Autodesk Inventor part; units mm, degrees
ref_plane "YZ Plane" through (0, 0, 0) normal (1, 0, 0) x (0, 1, 0)
ref_plane "XZ Plane" through (0, 0, 0) normal (0, 1, 0) x (-1, 0, 0)
ref_plane "XY Plane" through (0, 0, 0) normal (0, 0, 1) x (1, 0, 0)
sketch "Sketch1" plane through (0, 0, 0) normal (1, 0, 0) x (0, 1, 0)
  line L0 (24, 0) -> (64, 0)
  line L1 (64, 0) -> (64, 85)
  line L2 (64, 85) -> (24, 85)
  line L3 (24, -2) -> (24, 0)
  line L4 (24, 0) -> (24, 85)
  line L5 (24, 0) -> (109, 0) construction
  point P0 (0, 0)
  dimension "d1" = 85
  dimension "d13" = 90
extrude "Extrusion1" add sketch "Sketch1" along normal blind 2
sketch "Sketch2" plane through (2, 0, 0) normal (1, 0, 0) x (0, 0, -1)
  circle A0 centre (-75.4, 56) radius 1.85
  circle A1 centre (-75.4, 40) radius 1.85
  circle A2 centre (-9.6, 56) radius 1.85
  circle A3 centre (-9.6, 40) radius 1.85
  line L0 (-69, 24) -> (-69, 64)
  line L1 (-16, 24) -> (-16, 64)
  line L2 (-16, 0) -> (48, 0) construction
  line L3 (-85, 64) -> (-85, 24)
  line L4 (-69, 64) -> (-85, 64)
  line L5 (-85, 64) -> (-85, 24)
  line L6 (-69, 24) -> (-69, 64)
  line L7 (0, 24) -> (0, 64)
  line L8 (-16, 64) -> (0, 64)
  line L9 (0, 64) -> (0, 24)
  line L10 (-16, 24) -> (-16, 64)
  line L11 (-85, 24) -> (0, 24)
  point P0 (-69, 0)
  dimension "d5" = 90
extrude "Extrusion2" add sketch "Sketch2" along normal blind 3.2
chamfer "Chamfer1" distance 3.175 angle 45 2 edges at (2, 44, 16) (2, 44, 69)
sketch "Sketch3" plane through (5.2, 0, 0) normal (1, 0, 0) x (0, 0, -1)
  circle A0 centre (-75.4, 56) radius 1.85
  circle A1 centre (-75.4, 40) radius 1.85
  circle A2 centre (-9.6, 40) radius 1.85
  circle A3 centre (-9.6, 56) radius 1.85
  point P0 (0, 0)
extrude "Extrusion3" cut sketch "Sketch3" against normal through all
properties part number "wheelguard"
Can you work these out from the model? Positions are in its coordinate system, mm. A direction names the side the tool comes from. Give positions to 0.01 mm unless a question says otherwise; leave off trailing zeros. Write each loop counter-clockwise with the first axis right and the second up, starting at its lowest first coordinate (ties: lowest second). Pieces come first, ordered by that corner, then holes. Notation, with made-up numbers: (-29, 25) -> (25, 25) arc R11 ccw to (25, 36) -> close; hole circle Ø4 at (88, 19). An arc over 180 degrees is marked (long way). Write item = value, one per line.
(1) Suppose I cut it at A-A on x = 3.6. Write out the boundary of the cut face in (y, z) (3 decimals).
Worked out:
outline = (24, 0) -> (64, 0) -> (64, 17.575) -> (24, 17.575) -> close; (24, 67.425) -> (64, 67.425) -> (64, 85) -> (24, 85) -> close; hole circle Ø3.7 at (40, 9.6); hole circle Ø3.7 at (40, 75.4); hole circle Ø3.7 at (56, 9.6); hole circle Ø3.7 at (56, 75.4)
(2) Thinking about a two-plate mould opening in Z: for faces 1 (the face through (3, 44, 85)), 2 (the face through (0, 44, 43)), 3 (the face through (3.61, 43.72, 17.565)), which applies, released by +Z, released by -Z, zero draft, split by the parting line, or undercut?
Worked out:
face_1 = released by +Z
face_2 = zero draft
face_3 = undercut
(3) Suppose I cut it at C-C on y = 56. Write out the boundary of the cut face in (x, z) (3 decimals), then the cut area to 3 significant figures.
Worked out:
outline = (0, 0) -> (5.2, 0) -> (5.2, 7.75) -> (0, 7.75) -> close; (0, 11.45) -> (5.2, 11.45) -> (5.2, 16) -> (5.175, 16) -> (2, 19.175) -> (2, 65.825) -> (5.175, 69) -> (5.2, 69) -> (5.2, 73.55) -> (0, 73.55) -> close; (0, 77.25) -> (5.2, 77.25) -> (5.2, 85) -> (0, 85) -> close
area = 244 mm^2
(4) Suppose I cut it at B-B on z = 75.4. Write out the boundary of the cut face in (x, y), then the cut area to 3 significant figures.
Worked out:
outline = (0, 24) -> (5.2, 24) -> (5.2, 38.15) -> (0, 38.15) -> close; (0, 41.85) -> (5.2, 41.85) -> (5.2, 54.15) -> (0, 54.15) -> close; (0, 57.85) -> (5.2, 57.85) -> (5.2, 64) -> (0, 64) -> close
area = 170 mm^2
(5) I need wall thicknesses on probe 1 along Y at (x, z) = (3.7, 9.6); probe 2 along Z at (x, y) = (4.15, 41) (3 decimals); probe 3 along Z at (x, y) = (3.3, 55) (3 decimals). Which ranges of each line are inside material? Lowest first, please. Write a range as from..to.
Worked out:
probe_1 = 24..38.15, 41.85..54.15, 57.85..64
probe_2 = 0..8.044, 11.156..17.025, 67.975..73.844, 76.956..85
probe_3 = 0..8.044, 11.156..17.875, 67.125..73.844, 76.956..85
(6) Suppose I cut it at D-D on y = 45.5. Write out the boundary of the cut face in (x, z) (3 decimals), then the cut area to 3 significant figures.
Worked out:
outline = (0, 0) -> (5.2, 0) -> (5.2, 16) -> (5.175, 16) -> (2, 19.175) -> (2, 65.825) -> (5.175, 69) -> (5.2, 69) -> (5.2, 85) -> (0, 85) -> close
area = 282 mm^2
(7) For faces 4 (the face through (5.2, 44, 8)), 5 (the face through (2, 44, 43)), which set-ups out of +Z, -Z, +X, -X, +Y, -Y let a thin tool reach every point of the face, with its end or its side?
Worked out:
face_4 = +Z, -Z, +X, +Y, -Y
face_5 = +X, +Y, -Y
(8) I'm going to push flat-ended pins straight in: P1, Ø3, axis at y = 56, z = 75.4, coming from the -X side; P2, Ø12, axis at y = 38, z = 35, coming from the +X side. Where does each tip first touch, or does it pass through?
Worked out:
P1 = through
P2 = 2
